Design review of the part built by this model. Coordinates are the model's own, in mm. A direction names the side the tool comes from. Give positions to 0.01 mm unless a question says otherwise; leave off trailing zeros. Write each loop counter-clockwise with the first axis right and the second up, starting at its lowest first coordinate (ties: lowest second). Pieces come first, ordered by that corner, then holes.
```python
from build123d import *

# Parameters (mm, degrees)
SKETCH1_W           = 101.6
SKETCH1_H           = 44.45
BOSS_EXTRUDE1_DEPTH = 9.525
SKETCH2_W           = 88.9
SKETCH2_H           = 18.415
CUT_EXTRUDE1_DEPTH  = 10.525
FILLET1_R           = 5.08
SKETCH3_W           = 25.4
SKETCH3_H           = 25.4
CUT_EXTRUDE2_DEPTH  = 3.81
FILLET2_R           = 3.175
SKETCH4_R           = 1.5875
CUT_EXTRUDE3_DEPTH  = 10.525
SKETCH5_W           = 38.1
SKETCH5_H           = 7.62
CUT_EXTRUDE4_DEPTH  = 3.81


with BuildPart() as part:
    # Sketch1 → Boss-Extrude1 (new body)
    with BuildSketch(Plane(origin=(0, 0, 0), x_dir=(1, 0, 0), z_dir=(0, 1, 0))):
        Rectangle(SKETCH1_W, SKETCH1_H)
    extrude(amount=BOSS_EXTRUDE1_DEPTH)

    # Sketch2 → Cut-Extrude1 (cut, through all)
    with BuildSketch(Plane(origin=(0, 9.525, 0), x_dir=(1, 0, 0), z_dir=(0, 1, 0))):
        with Locations((0, -13.0175)):
            Rectangle(SKETCH2_W, SKETCH2_H)
    cut_extrude1 = extrude(amount=-CUT_EXTRUDE1_DEPTH, mode=Mode.SUBTRACT)

    # Mirror1: Cut-Extrude1 across plane
    add(cut_extrude1.mirror(Plane.XY), mode=Mode.SUBTRACT)

    # Fillet1
    fillet1_edges = [part.edges().sort_by_distance(p)[0] for p in [
        (-44.45, 4.7625, 3.81),
        (44.45, 4.7625, 3.81),
        (-44.45, 4.7625, -3.81),
        (44.45, 4.7625, -3.81),
    ]]
    fillet(fillet1_edges, radius=FILLET1_R)

    # Sketch3 → Cut-Extrude2 (cut)
    with BuildSketch(Plane(origin=(0, 9.525, 0), x_dir=(1, 0, 0), z_dir=(0, 1, 0))):
        with Locations((-38.1, 0)):
            Rectangle(SKETCH3_W, SKETCH3_H)
    cut_extrude2 = extrude(amount=-CUT_EXTRUDE2_DEPTH, mode=Mode.SUBTRACT)

    # Mirror2: Cut-Extrude2 across plane
    add(cut_extrude2.mirror(Plane(origin=(0, 0, 0), x_dir=(0, 0, 1), z_dir=(1, 0, 0))), mode=Mode.SUBTRACT)

    # Fillet2
    fillet2_edges = [part.edges().sort_by_distance(p)[0] for p in [
        (47.625, 5.715, -12.7),
        (47.625, 5.715, 12.7),
        (25.4, 5.715, 0),
        (-47.625, 5.715, 12.7),
        (-25.4, 5.715, 0),
        (-47.625, 5.715, -12.7),
    ]]
    fillet(fillet2_edges, radius=FILLET2_R)

    # Sketch4 → Cut-Extrude3 (cut, through all)
    with BuildSketch(Plane.XZ):
        with Locations((-12.7, 0)):
            Circle(SKETCH4_R)
    cut_extrude3 = extrude(amount=-CUT_EXTRUDE3_DEPTH, mode=Mode.SUBTRACT)

    # Sketch5 → Cut-Extrude4 (cut)
    with BuildSketch(Plane.XZ):
        Rectangle(SKETCH5_W, SKETCH5_H)
    extrude(amount=-CUT_EXTRUDE4_DEPTH, mode=Mode.SUBTRACT)

    # Mirror3: Cut-Extrude3 across plane
    add(cut_extrude3.mirror(Plane(origin=(0, 0, 0), x_dir=(0, 0, 1), z_dir=(1, 0, 0))), mode=Mode.SUBTRACT)


solid = part.part
```
(1) Clearance check with flat-ended pins moving along their axes: P1, Ø1.5, axis at x = 21, y = 2, coming from the +Z side; P2, Ø5, axis at x = 18.5, y = 7, coming from the -Z side; P3, Ø8.5, axis at x = 8.5, z = 1, coming from the -Y side. State where each tip first meets the part, or that it passes through.
Resolved:
P1: stops at z = 3.81
P2: stops at z = -3.81
P3: stops at y = 3.81
(2) Consider section D-D, the plane x = 23.5. Give the boundary of the cut face in (y, z) (3 decimals), then the cut area to 3 significant figures.
Resolved:
outline: (0, -3.81) - (9.525, -3.81) - (9.525, 3.81) - (0, 3.81) - close
area: 72.6 mm2
(3) Tool access review of faces 4 (the face through (-44.45, 5, 16)), 5 (the face through (-42, 5.715, 0)), 6 (the face through (42, 5.715, 0)): name each direction out of +Z, -Z, +X, -X, +Y, -Y from which nothing blocks a thin tool from reaching the whole face with its end or side.
Resolved:
face 4: +Z, +Y, -Y
face 5: -X, +Y
face 6: +X, +Y
(4) To check wall thickness, follow L1, parallel to Z at x = -12.7, y = 6.1; L2, parallel to X at y = 0.5, z = -13; L3, parallel to Z at x = -8, y = 4.25. State the ranges of each line that lie inside material, in increasing order.
Resolved:
L1: z = -3.81 to -1.59, 1.59 to 3.81
L2: x = -50.8 to -44.45, 44.45 to 50.8
L3: z = -3.81 to 3.81
(5) Mouldability with a two-part tool opening along X and no side actions: class faces 1 (the face through (47.581, 6.62, -11.745)), 2 (the face through (0, 3.81, 0)), 3 (the face through (-26.355, 6.62, -0.053)) as pulls with the +X half, pulls with the -X half, needs draft (parallel to the pull), parting line crosses it, or undercut.
Resolved:
face 1: needs draft
face 2: undercut
face 3: pulls with the -X half
(6) Consider section A-A, the plane x = -12.7. Give the boundary of the cut face in (y, z) (1 decimal).
Resolved:
outline: (3.8, -3.8) - (9.5, -3.8) - (9.5, -1.6) - (3.8, -1.6) - close; (3.8, 1.6) - (9.5, 1.6) - (9.5, 3.8) - (3.8, 3.8) - close
(7) Consider section B-B, the plane y = 4.75. Give the number of separate pieces and of enclosed holes in the cut face, then the cut area to 3 significant figures.
Resolved:
separate pieces: 1
enclosed holes: 2
area: 1,250 mm2
